Autodesk Inventor part; units mm, degrees
ref_plane "YZ Plane" through (0, 0, 0) normal (1, 0, 0) x (0, 1, 0)
ref_plane "XZ Plane" through (0, 0, 0) normal (0, 1, 0) x (-1, 0, 0)
ref_plane "XY Plane" through (0, 0, 0) normal (0, 0, 1) x (1, 0, 0)
sketch "Sketch1" plane through (0, 0, 0) normal (1, 0, 0) x (0, 1, 0)
  line L0 (0, 0) -> (0, -44.45)
  line L1 (0, 0) -> (57.15, 0)
  line L2 (0, -44.45) -> (6.35, -44.45)
  line L3 (6.35, -44.45) -> (23.495, -21.59)
  line L4 (57.15, 0) -> (76.2, 0)
  line L5 (76.2, 0) -> (76.2, -12.7)
  line L6 (76.2, -12.7) -> (57.15, -12.7)
  line L7 (57.15, -12.7) -> (57.15, -44.45)
  line L8 (57.15, -44.45) -> (50.8, -44.45)
  line L9 (50.8, -44.45) -> (33.655, -21.59)
  arc A0 (33.655, -21.59) -> (23.495, -21.59) centre (28.575, -25.4) ccw
  point P0 (28.575, -14.8167)
  dimension "d36" = 44.45
  dimension "d37" = 57.15
  dimension "d38" = 6.35
  dimension "d40" = 28.575
  dimension "d41" = 19.05
  dimension "d42" = 12.7
  dimension "d43" = 44.45
  dimension "d44" = 57.15
  dimension "d48" = 6.35
  dimension "d53" = 19.05
revolve "Revolution1" add sketch "Sketch1" angle 360 about axis through (0, 0, 0) along (0, 1, 0)
sketch "Sketch6" plane through (0, 76.2, 0) normal (0, 1, 0) x (1, 0, 0)
  line L0 (7.6623, 0) -> (3.8312, -6.6357)
  line L1 (3.8312, -6.6357) -> (-3.8312, -6.6357)
  line L2 (-3.8312, -6.6357) -> (-7.6623, 0)
  line L3 (-7.6623, 0) -> (-3.8312, 6.6357)
  line L4 (-3.8312, 6.6357) -> (3.8312, 6.6358)
  line L5 (3.8312, 6.6358) -> (7.6623, 0)
  point P0 (0, 0)
  point P1 (0, 0)
  dimension "d45" = 13.2715
extrude "Extrusion5" cut sketch "Sketch6" against normal through all
chamfer "Chamfer4" distance 1.5875 angle 45 12 edges at (5.7467, 76.2, 3.3179) (5.7467, 76.2, -3.3179) (0, 76.2, -6.6358) (-5.7467, 76.2, -3.3179) (-5.7467, 76.2, 3.3179) (0, 76.2, 6.6357) (-5.7467, 0, -3.3179) (0, 0, -6.6358) (5.7467, 0, -3.3179) (5.7467, 0, 3.3179) (0, 0, 6.6357) (-5.7467, 0, 3.3179)
fillet "Fillet1" radius 6.35 2 edges at (0, 50.8, 44.45) (0, 6.35, 44.45)
equation "\"d36\" = spoolExteriorRadius"
equation "\"d37\" = spoolHeight"
equation "\"d38\" = supportChannels"
equation "\"d41\" = spacerHeight"
equation "\"d43\" = spoolExteriorRadius"
equation "\"d44\" = spoolHeight"
equation "\"d53\" = spoolInteriroRadius"
equation "\"d45\" = hexDiameter"
equation "\"d49\" = hexHoleChamfer"
equation "\"holeForString\" = stringDiameter + clearanceForString"
equation "\"stringDiameter\" = 3"
equation "\"clearanceForString\" = 0.5"
equation "\"spoolHeight\" = 57.15"
equation "\"hexShaftDiameter\" = 12.7"
equation "\"clearanceForHexShaft\" = 0.5715"
equation "\"hexDiameter\" = hexShaftDiameter + clearanceForHexShaft"
equation "\"supportChannels\" = 6.35"
equation "\"spoolInteriorDiameter\" = 38.1"
equation "\"spoolInteriroRadius\" = 0.5 * spoolInteriorDiameter"
equation "\"spoolExteriorDiameter\" = 88.9"
equation "\"spoolExteriorRadius\" = 0.5 * spoolExteriorDiameter"
equation "\"spoolFiletRadius\" = 0.5 * supportChannels"
equation "\"holeCenter\" = 0.25 * spoolHeight - 0.75 * supportChannels"
equation "\"hexHoleChamfer\" = 1.5875"
equation "\"stringHoleCenterFromHexShaft\" = 0.5 * hexDiameter + 0.5 * holeForString"
equation "\"textCircleDiameter\" = 0.75 * spoolExteriorDiameter"
equation "\"textHeight\" = 6.096"
equation "\"textDepth\" = 1.27"
equation "\"stringHoleChamfer\" = 1.5875"
equation "\"halfSpoolHeight\" = 0.5 * spoolHeight"
equation "\"spoolTotalHeight\" = 76.2"
equation "\"spacerHeight\" = spoolTotalHeight - spoolHeight"
properties part number "spoolV02"
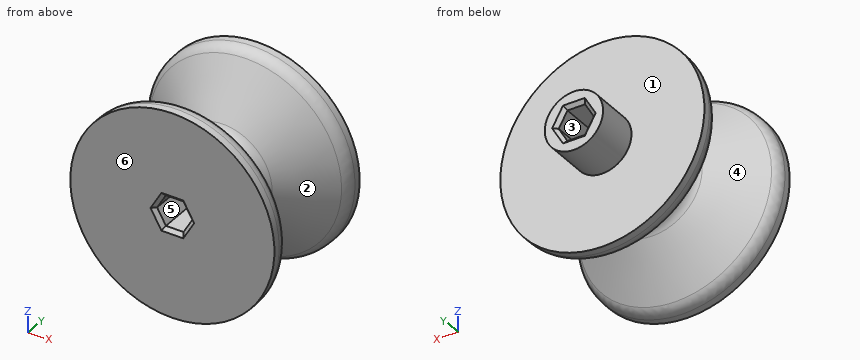
Model file for the job. Use its own axes, mm. Face numbers are marked on the shaded views. A direction names the side the tool comes from. Give positions to 0.01 mm unless a question says otherwise; leave off trailing zeros. Loops run counter-clockwise (first coordinate to the right, second up) from the corner with the lowest first, then second, coordinate; pieces in that order, holes last. Notation, with made-up numbers: (75.5, 16.25) -> (111.5, 16.25) arc R13 cw to (111.5, 36.25) -> close; hole circle Ø10 at (55.25, 11.5). An arc over 180 degrees is marked (long way). Use CSV: the item, a comma, the result in double quotes. Start each with the question number.
1) Slice it at A-A on y = 9.5. Give the cut face in (x, z).
2) Mould opens along X. For the marked faces 4, 5 and 6 say: released by +X, released by -X, zero draft, split by the parting line, or undercut.
3) Flat gauge pins, fed straight in: pin 1 Ø1 at (x, y) = (-9.5, 48) entering from -Z; pin 2 Ø6 at (x, y) = (-1, 40) entering from +Z; pin 3 Ø1.5 at (x, z) = (12, -21.5) entering from +Y. Where does each tip first touch, or does it go through?
4) Tool access for the marked faces 1, 2 and 3: list every direction of +Z, -Z, +X, -X, +Y, -Y with a clear straight run to the whole face (end or side of a thin tool).
5) Wall check: line 1 (Y direction, x = -19, z = -35.5); line 2 (X direction, y = 62, z = 5); line 3 (Z direction, x = -7, y = 65). Give the ranges that are in metal, low to high.
Computed values:
1,outline,"circle Ø80.5 at (0, 0); hole (-7.66, 0) -> (-3.83, -6.64) -> (3.83, -6.64) -> (7.66, 0) -> (3.83, 6.64) -> (-3.83, 6.64) -> close"
2,face 4,"split by the parting line"
2,face 5,"undercut"
2,face 6,"zero draft"
3,pin 1,"stops at z = -40.29"
3,pin 2,"stops at z = 34.04"
3,pin 3,"stops at y = 57.15"
4,face 1,"+Y"
4,face 2,"none"
4,face 3,"+Y, -Y"
5,line 1,"y = 0 to 9.49, 47.66 to 57.15"
5,line 2,"x = -11.67 to -4.78, 4.78 to 11.67"
5,line 3,"z = -10.6 to -1.15, 1.15 to 10.6"
